```python
from build123d import *

# Parameters (mm, degrees)
F0_R     = 12.5
F1_DEPTH = 2
F2_R     = 1
F3_R     = 2.5
F4_DEPTH = 25.4


with BuildPart() as f1:
    # F0 (on Top) → F1 (new body)
    with BuildSketch(Plane.XY):
        Circle(F0_R)
    extrude(amount=F1_DEPTH)

    # F2
    f2_edges = [f1.edges().sort_by_distance(p)[0] for p in [
        (-12.5, 0, 2),
    ]]
    fillet(f2_edges, radius=F2_R)

    # F3 (on face) → F4 (cut)
    with BuildSketch(Plane(origin=(0, 0, 0), x_dir=(1, 0, 0), z_dir=(0, 0, -1))):
        Circle(F3_R)
    extrude(amount=-F4_DEPTH, mode=Mode.SUBTRACT)


solid = f1.part
```
The model under review builds one solid part; all positions refer to its coordinate system, in mm. Round coordinates to 2 decimals unless told otherwise and drop trailing zeros. Order: outer loops, then holes, each group sorted by start corner. A loop starts at its lowest first (then second) coordinate and runs counter-clockwise, first axis right, second up. Notation, with made-up numbers: (76.25, 11.5) - (109.25, 11.5) arc R16 ccw to (109.25, 30.5) - close; hole circle Ø9 at (-25, 4). An arc over 180 degrees is marked (long way). Answer in a Markdown table with one row per item.
(1) Mouldability with a two-part tool opening along X and no side actions: class faces 1 (the face through (-3, 0, 2)), 2 (the face through (11.923, 3.755, 0.493)), 3 (the face through (-0.54, 2.44, 0.99)) as released by +X, released by -X, zero draft, split by the parting line, or undercut.
Result set:
| item | result |
|---|---|
| face 1 | zero draft |
| face 2 | split by the parting line |
| face 3 | undercut |
(2) For line 1 (Y direction, x = 0, z = 0.75); line 2 (X direction, y = 1, z = 1.8); line 3 (Y direction, x = -2, z = 0.5), list the stretches that pass through material, from the lowest coordinate up. Write a range as from..to.
Result set:
| item | result |
|---|---|
| line 1 | y = -12.5..-2.5, 2.5..12.5 |
| line 2 | x = -12.06..-2.29, 2.29..12.06 |
| line 3 | y = -12.34..-1.5, 1.5..12.34 |
(3) Clearance check with flat-ended pins moving along their axes: P1, Ø1, axis at x = 8, z = 1, coming from the +Y side; P2, Ø4.5, axis at x = 0, y = 0, coming from the -Z side. State where each tip first meets the part, or that it passes through.
Result set:
| item | result |
|---|---|
| P1 | stops at y = 10 |
| P2 | passes through |
(4) Take a section at A-A on y = 0. Write out the cut boundary in (x, z).
Result set:
| item | result |
|---|---|
| outline | (-12.5, 0) - (-2.5, 0) - (-2.5, 2) - (-11.5, 2) arc R1 ccw to (-12.5, 1) - close; (2.5, 0) - (12.5, 0) - (12.5, 1) arc R1 ccw to (11.5, 2) - (2.5, 2) - close |
(5) Take a section at C-C on z = 0.6. Write out the cut boundary in (x, y).
Result set:
| item | result |
|---|---|
| outline | circle Ø25 at (0, 0); hole circle Ø5 at (0, 0) |
